```python
from build123d import *

# Parameters (mm, degrees)
F1_DEPTH = 5
F2_W     = 15.590731
F2_H     = 24.653931
F3_DEPTH = 4
F4_DEPTH = 3
F5_DEPTH = 2
F6_DEPTH = 1


with BuildPart() as f1:
    # F0 (on Front) → F1 (new body)
    with BuildSketch(Plane.XZ):
        with BuildLine():
            Line((-37.5, -23.5), (37.5, -23.5))
            ThreePointArc((37.5, -23.5), (41.035534, -22.035534), (42.5, -18.5))
            Line((42.5, -18.5), (42.5, 18.5))
            ThreePointArc((42.5, 18.5), (41.035534, 22.035534), (37.5, 23.5))
            Line((37.5, 23.5), (-37.5, 23.5))
            ThreePointArc((-37.5, 23.5), (-41.035534, 22.035534), (-42.5, 18.5))
            Line((-42.5, 18.5), (-42.5, -18.5))
            ThreePointArc((-42.5, -18.5), (-41.035534, -22.035534), (-37.5, -23.5))
        make_face()
    extrude(amount=F1_DEPTH)

    # F2 (on face) → F3 (cut)
    with BuildSketch(Plane.XZ.offset(5)):
        with Locations((-29.650416, -5.826966)):
            Rectangle(F2_W, F2_H)
    extrude(amount=-F3_DEPTH, mode=Mode.SUBTRACT)

    # F2 (on face) → F4 (cut)
    with BuildSketch(Plane.XZ.offset(5)):
        with Locations((-9.850416, -5.826966)):
            Rectangle(F2_W, F2_H)
    extrude(amount=-F4_DEPTH, mode=Mode.SUBTRACT)

    # F2 (on face) → F5 (cut)
    with BuildSketch(Plane.XZ.offset(5)):
        with Locations((9.949583, -5.826966)):
            Rectangle(F2_W, F2_H)
    extrude(amount=-F5_DEPTH, mode=Mode.SUBTRACT)

    # F2 (on face) → F6 (cut)
    with BuildSketch(Plane.XZ.offset(5)):
        with Locations((29.749583, -5.826966)):
            Rectangle(F2_W, F2_H)
    extrude(amount=-F6_DEPTH, mode=Mode.SUBTRACT)


solid = f1.part
```
The listing builds one solid part. Answer for the finished solid, in the listing's coordinates (mm). A direction names the side the tool comes from. Coordinates: 2 decimals unless noted, no trailing zeros. Loops run counter-clockwise (first coordinate to the right, second up) from the corner with the lowest first, then second, coordinate; pieces in that order, holes last. Notation, with made-up numbers: (-1.75, 53.5) -> (3.25, 53.5) arc R12 cw to (3.25, 64.5) -> close; hole circle Ø11 at (63.5, 1). An arc over 180 degrees is marked (long way). Use one line per item in the form item = value. Start each with the question number.
Item 1: The part is cut by section B-B on z = -2. Determine the outline of the cut face in (x, y).
Item 2: The part is cut by section A-A on x = 26. Determine the outline of the cut face in (y, z), then the cut area to 3 significant figures.
Item 3: Flat-ended cylindrical pins translate along their axes: pin 1 Ø2 at (x, z) = (28, -2.5) entering from -Y; pin 2 Ø1.5 at (x, z) = (16.5, -6.5) entering from -Y. Find the tip coordinate at first contact, or state that the pin passes through.
Item 4: Consider L1, parallel to X at y = -3.55, z = -16; L2, parallel to X at y = -2.2, z = -8; L3, parallel to Z at x = -36.5, y = -2.75. Determine where each line is inside the solid, lowest interval first. Write a range as [from, to].
Item 5: The mould has two halves that part along Z. Classify faces 3 (the face through (1, -2, 23.5)), 4 (the face through (-30, -1, -6)), 5 (the face through (-1, 0, 0)): released by +Z, released by -Z, zero draft, split by the parting line, or undercut.
Item 6: The part is cut by section C-C on x = -24. Determine the outline of the cut face in (y, z).
Item 7: A tool of negligible diameter and unlimited length cuts with its end or side. For faces 1 (the face through (-37.446, -3, -6)), 2 (the face through (-1, -2, -23.5)), from which of +Z, -Z, +X, -X, +Y, -Y can it reach the whole face along a straight path? Write none if from no direction.
Answer key:
q1.outline = (-42.5, -5) -> (-37.45, -5) -> (-37.45, -1) -> (-21.86, -1) -> (-21.86, -5) -> (-17.65, -5) -> (-17.65, -2) -> (-2.06, -2) -> (-2.06, -5) -> (2.15, -5) -> (2.15, -3) -> (17.74, -3) -> (17.74, -5) -> (21.95, -5) -> (21.95, -4) -> (37.54, -4) -> (37.54, -5) -> (42.5, -5) -> (42.5, 0) -> (-42.5, 0) -> close
q2.outline = (-5, -23.5) -> (0, -23.5) -> (0, 23.5) -> (-5, 23.5) -> (-5, 6.5) -> (-4, 6.5) -> (-4, -18.15) -> (-5, -18.15) -> close
q2.area = 210 mm2
q3.pin_1 = -4
q3.pin_2 = -3
q4.L1 = [-42.5, -37.45], [-21.86, -17.65], [-2.06, 2.15], [17.74, 42.5]
q4.L2 = [-42.5, -37.45], [-21.86, -17.65], [-2.06, 42.5]
q4.L3 = [-23.5, -18.15], [6.5, 23.5]
q5.face_3 = released by +Z
q5.face_4 = undercut
q5.face_5 = zero draft
q6.outline = (-5, -23.5) -> (0, -23.5) -> (0, 23.5) -> (-5, 23.5) -> (-5, 6.5) -> (-1, 6.5) -> (-1, -18.15) -> (-5, -18.15) -> close
q7.face_1 = -Y
q7.face_2 = -Z, +X, -X, +Y, -Y
